Geometry: final body of the model. Coordinates: model frame, mm. A direction names the side the tool comes from. Give positions to 0.01 mm unless a question says otherwise; leave off trailing zeros. Answer as a JSON object with one key per item and string values.
from build123d import *

# Parameters (mm, degrees)
F3_D     = 2.7178
F3_DEPTH = 11.176
F3_TIP   = 0.8165094952
F2_R     = 1.7526
F4_DEPTH = 7.112
F8_DEPTH = 1.5748
F9_R     = 1.524


with BuildPart() as f1:
    # F0 (on Front) → F1 (revolve)
    with BuildSketch(Plane.XZ):
        with BuildLine():
            ThreePointArc((35.941, 17.3736), (19.2278, 21.4249124266), (2.5146, 17.3736))
            Line((2.5146, 17.3736), (0, 17.3736))
            Line((0, 17.3736), (0, 9.525))
            Line((0, 9.525), (3.175, 9.525))
            Line((3.175, 9.525), (3.175, 6.35))
            Line((3.175, 6.35), (5.715, 6.35))
            Line((5.715, 6.35), (7.5480871047, 9.525))
            Line((7.5480871047, 9.525), (114.3, 9.525))
            Line((114.3, 9.525), (114.3, 14.2875))
            Line((114.3, 14.2875), (35.941, 14.2875))
            Line((35.941, 14.2875), (35.941, 17.3736))
        make_face()
    revolve(axis=Axis((57.15, 0, 0), (1, 0, 0)))

    # F3
    with Locations(Plane(origin=(0, 0, 0), x_dir=(0, -1, 0), z_dir=(-1, 0, 0))):
        with Locations((-13.5001, 0), (0, 13.4874), (13.5001, 0)):
            Hole(F3_D / 2, depth=F3_DEPTH)
            with Locations((0, 0, -(F3_DEPTH + F3_TIP / 2))):  # 118° drill point
                Cone(0, F3_D / 2, F3_TIP, mode=Mode.SUBTRACT)

    # F2 (on face) → F4 (cut)
    with BuildSketch(Plane(origin=(0, 0, 0), x_dir=(0, -1, 0), z_dir=(-1, 0, 0))):
        with Locations((-13.5001, 0)):
            Circle(F2_R)
        with Locations((0, 13.4874)):
            Circle(F2_R)
        with Locations((13.5001, 0)):
            Circle(F2_R)
    extrude(amount=-F4_DEPTH, mode=Mode.SUBTRACT)

    # F7 (on plane+point) → F8 (cut)
    with BuildSketch(Plane.XY.offset(-14.2875)):
        with BuildLine():
            Line((55.8546, -3.175), (114.3, -3.175))
            Line((114.3, -3.175), (114.3, 3.175))
            Line((114.3, 3.175), (55.8546, 3.175))
            ThreePointArc((55.8546, 3.175), (52.6796, 0), (55.8546, -3.175))
        make_face()
    extrude(amount=F8_DEPTH, mode=Mode.SUBTRACT)

    # F9
    f9_edges = [f1.edges().sort_by_distance(p)[0] for p in [
        (35.941, 0, -14.2875),
    ]]
    fillet(f9_edges, radius=F9_R)


solid = f1.part
1) Contact query for flat-ended pins moving along their axis: P1, Ø3, axis at y = 0, z = 13.49, coming from the -X side; P2, Ø3, axis at x = 86.5, y = 0.5, coming from the -Z side; P3, Ø2, axis at y = -13.5, z = 0, coming from the -X side. Output: stop coordinate, or through.
Geometry check:
{"P1": "stops at x = 7.11", "P2": "stops at z = -12.71", "P3": "stops at x = 11.39"}
2) Pull-direction query (Y, two-part tool) for faces 6 (the cylindrical face through (75.34, -4.29, 13.63)), 7 (the cylindrical face through (3.506, 0.228, 15.225)), 8 (the flat face through (114.3, -10, 0)); classes: pulls with the +Y half, pulls with the -Y half, needs draft (parallel to the pull), parting line crosses it, or undercut.
Geometry check:
{"face 6": "parting line crosses it", "face 7": "undercut", "face 8": "needs draft"}
3) Line query: line 1 (Y direction, x = 10, z = 0) (3 decimals); line 2 (Z direction, x = 4.45, y = 0); line 3 (Z direction, x = 5.75, y = 0). Output: solid intervals per line, ascending. Write a range as from..to.
Geometry check:
{"line 1": "y = -20.239..-14.859, -12.141..-9.525, 9.525..12.141, 14.859..20.239", "line 2": "z = -18.3..-6.35, 6.35..11.73, 15.24..18.3", "line 3": "z = -18.85..-6.41, 6.41..11.73, 15.24..18.85"}
4) Set-up query: faces 1 (the cylindrical face through (4.46, 6.2, -1.38)), 2 (the cylindrical face through (61.671, 5.796, -7.559)), 3 (the flat face through (83, 0, -12.713)), 4 (the flat face through (0, 7, 7)), 5 (the cylindrical face through (9.172, 14.755, -0.52)). Return all of +Z, -Z, +X, -X, +Y, -Y with unobstructed straight access to the full face (end or side cutting, diameter ignored); none if empty.
Geometry check:
{"face 1": "+X, -X", "face 2": "+X", "face 3": "-Z, +X", "face 4": "+Z, -Z, -X, +Y, -Y", "face 5": "-X"}
